Read the model definition and answer for the solid it produces. Units are mm, in the model's axes. A direction names the side the tool comes from. Give positions to 0.01 mm unless a question says otherwise; leave off trailing zeros. Order: outer loops, then holes, each group sorted by start corner. A loop starts at its lowest first (then second) coordinate and runs counter-clockwise, first axis right, second up. Notation, with made-up numbers: (22, 75.25) - (52, 75.25) arc R10 ccw to (52, 87.25) - close; hole circle Ø9 at (74.5, 77). An arc over 180 degrees is marked (long way). Write each question's results on one line, items separated by ' | '.
Autodesk Inventor part; units mm, degrees
ref_plane "Work Plane1" through (0, -27.5, 0) normal (1, 0, 0) x (0, 0, -1)
ref_plane "Work Plane2" through (-48.55, 0, 0) normal (0, 1, 0) x (1, 0, 0)
ref_plane "YZ Plane" through (0, 0, 0) normal (1, 0, 0) x (0, 1, 0)
sketch "Sketch1" plane through (0, 0, 0) normal (0, 0, 1) x (1, 0, 0)
  line L0 (-60, -27.5) -> (60, -27.5)
  line L1 (60, -27.5) -> (60, 27.5)
  line L2 (60, 27.5) -> (-60, 27.5)
  line L3 (-60, 27.5) -> (-60, -27.5)
  line L4 (-60, -27.5) -> (60, 27.5) construction
  line L5 (60, -27.5) -> (-60, 27.5) construction
  point P0 (0, 0)
  dimension "d0" = 120
  dimension "d1" = 55
extrude "Extrusion1" add sketch "Sketch1" against normal blind 4
sketch "Sketch2" plane through (60, -27.5, 0) normal (1, 0, 0) x (0, 0, -1)
  circle A0 centre (2, 2) radius 2
  line L0 (0, 0) -> (4, 0)
  line L1 (4, 55) -> (4, 0)
  circle A1 centre (2, 2) radius 1.25
  circle A2 centre (2, 53) radius 2
  line L2 (0, 55) -> (4, 55)
  circle A3 centre (2, 53) radius 1.25
  line L3 (0, 55) -> (0, 0)
  line L4 (0, 55) -> (4, 55)
  line L5 (4, 55) -> (4, 0)
  line L6 (4, 0) -> (0, 0)
  line L7 (0, 0) -> (0, 55)
  point P0 (0, 27.5)
  dimension "d4" = 4
  dimension "d5" = 2.5
  dimension "d6" = 4
  dimension "d7" = 2.5
extrude "Extrusion2" cut sketch "Sketch2" against normal blind 3.5 contours L1 L0 A0 | A0 L3 A2 L1 | A0 L0 L3 | A2 L2 L1 | L3 L2 A2
extrude "Extrusion3" cut sketch "Sketch2" against normal blind 25 contours A1
extrude "Extrusion4" cut sketch "Sketch2" against normal blind 25 contours A3
sketch "Sketch3" plane through (-60, -27.5, 0) normal (-1, 0, 0) x (0, 0, 1)
  circle A0 centre (-2, 2) radius 2
  circle A1 centre (-2, 53) radius 2
  line L0 (0, 0) -> (-4, 0)
  line L1 (-4, 0) -> (-4, 55)
  line L2 (0, 55) -> (-4, 55)
  line L3 (0, 55) -> (0, 0)
  line L4 (-4, 0) -> (0, 0)
  line L5 (0, 0) -> (0, 55)
  line L6 (0, 55) -> (-4, 55)
  line L7 (-4, 55) -> (-4, 0)
  circle A2 centre (-2, 2) radius 1.25
  circle A3 centre (-2, 2) radius 1.25
  circle A4 centre (-2, 53) radius 1.25
  circle A5 centre (-2, 53) radius 1.25
  point P0 (0, 27.5)
  dimension "d14" = 4
  dimension "d15" = 4
  dimension "d16" = 2.5
  dimension "d17" = 2.5
extrude "Extrusion5" cut sketch "Sketch3" against normal blind 3.5 contours L3 L0 A0 | A0 L1 A1 L3 | A0 L0 L1 | A1 L2 L3 | L1 L2 A1
extrude "Extrusion6" cut sketch "Sketch3" against normal blind 25 contours A4
extrude "Extrusion7" cut sketch "Sketch3" against normal blind 25 contours A2
sketch "Sketch4" plane through (0, 0, 0) normal (0, 0, 1) x (1, 0, 0)
  line L0 (-56.5, 27.5) -> (56.5, 27.5)
  line L1 (56.5, -27.5) -> (-56.5, -27.5)
  line L2 (-56.5, 27.5) -> (56.5, 27.5)
  line L3 (56.5, 27.5) -> (56.5, -27.5)
  line L4 (56.5, -27.5) -> (-56.5, -27.5)
  line L5 (-56.5, -27.5) -> (-56.5, 27.5)
  line L6 (-73.441, 25.5) -> (75.6749, 25.5) construction
  line L7 (-49.5, 37.9771) -> (-49.5, -42.6684) construction
  line L8 (-50.45, 28) -> (-48.55, 28)
  line L9 (-48.55, 28) -> (-48.55, 23)
  line L10 (-48.55, 23) -> (-50.45, 23)
  line L11 (-50.45, 23) -> (-50.45, 28)
  line L12 (-50.45, 28) -> (-48.55, 23) construction
  line L13 (-48.55, 28) -> (-50.45, 23) construction
  point P0 (0, 0)
  point P1 (-49.5, 25.5)
  dimension "d24" = 2
  dimension "d25" = 7
  dimension "d26" = 1.9
  dimension "d27" = 5
extrude "Extrusion8" cut sketch "Sketch4" against normal blind 25 contours L11 L8 L9 L0 | L0 L9 L10 L11
ref_plane "Work Plane1" through (0, -27.5, 0) normal (1, 0, 0) x (0, 0, -1)
ref_plane "Work Plane2" through (-48.55, 0, 0) normal (0, 1, 0) x (1, 0, 0)
mirror "Mirror1" about plane through (0, -27.5, 0) normal (1, 0, 0) of "Extrusion8"
mirror "Mirror3" about plane through (-48.55, 0, 0) normal (0, 1, 0) of "Extrusion8", "Mirror1"
sketch "Sketch5" plane through (0, 0, 0) normal (0, 0, 1) x (1, 0, 0)
  line L0 (-20.311, 26.3647) -> (47.689, 26.3647) construction
  line L1 (47.689, 26.3647) -> (47.689, -26.6353) construction
  line L2 (47.689, -26.6353) -> (-20.311, -26.6353) construction
  line L3 (-20.311, -26.6353) -> (-20.311, 26.3647) construction
  line L4 (34.689, 35.6432) -> (34.689, -53.7477) construction
  line L5 (-67.7221, 24) -> (59.2356, 24) construction
  line L6 (-64.2143, -24) -> (60.4803, -24) construction
  line L7 (-93.3625, 0) -> (86.1208, 0) construction
  circle A0 centre (34.689, 24) radius 2.5
  circle A1 centre (34.689, -24) radius 2.5
  line L8 (-15.0696, 19.4646) -> (-13.0566, 19.4646)
  line L9 (-13.0566, 19.4646) -> (-13.0566, -11.8201)
  line L10 (-13.0566, -11.8201) -> (-15.0696, -11.8201)
  line L11 (-15.0696, -11.8201) -> (-15.0696, 19.4646)
  circle A2 centre (34.689, 24) radius 0.75
  circle A3 centre (34.689, -24) radius 0.75
  point P0 (0, 0)
  dimension "d30" = 68
  dimension "d31" = 53
  dimension "d32" = 13
  dimension "d34" = 48
  dimension "d35" = 24
  dimension "d36" = 5
  dimension "d37" = 5
  dimension "d42" = 1.5
  dimension "d43" = 1.5
extrude "Extrusion9" add sketch "Sketch5" along normal blind 4 contours A0 | A1 | A2 | A3
extrude "Extrusion10" add sketch "Sketch5" along normal blind 4 contours L8 L9 L10 L11
sketch "Sketch6" plane through (34.689, 24, 4) normal (0, 0, 1) x (1, 0, 0)
  circle A0 centre (0, 0) radius 0.75
  circle A1 centre (0, -48.0486) radius 0.75
  point P0 (-34.689, -24)
  dimension "d44" = 1.5
  dimension "d45" = 1.5
extrude "Extrusion11" cut sketch "Sketch6" against normal blind 7
sketch "Sketch7" plane through (0, 0, 0) normal (0, 0, 1) x (1, 0, 0)
  line L0 (-56.5, -25.5) -> (-56.5, 25.5)
  line L1 (-56.5, 20) -> (-16.5, 20)
  line L2 (-16.5, 20) -> (-16.5, -20)
  line L3 (-16.5, -20) -> (-56.5, -20)
  line L4 (-56.5, -20) -> (-56.5, 20)
  line L5 (48.55, 27.5) -> (-48.55, 27.5)
  line L6 (-8.902, 20) -> (51.098, 20)
  line L7 (51.098, 20) -> (51.098, -20)
  line L8 (51.098, -20) -> (-8.902, -20)
  line L9 (-8.902, -20) -> (-8.902, 20)
  point P0 (0, 0)
  dimension "d48" = 40
  dimension "d49" = 40
  dimension "d50" = 7.5
  dimension "d51" = 60
extrude "Extrusion12" cut sketch "Sketch7" against normal blind 7
fillet "Fillet1" radius 2 6 edges at (-16.5, -20, -2) (-16.5, 20, -2) (-8.902, 20, -2) (-8.902, -20, -2) (51.098, 20, -2) (51.098, -20, -2)
properties part number "Drivercarrier"
(1) Each of these flat-tipped pins is pushed along its axis until it touches: pin 1 (1.2 mm diameter, centred on y = -8, z = -1.5, fed in from -X); pin 2 (2 mm diameter, centred on y = 2.5, z = 1.5, fed in from +X); pin 3 (2 mm diameter, centred on y = -8, z = -2, fed in from +X). Where does it stop, or does it pass through?
Conclusion:
pin 1: x = -16.5 | pin 2: x = -13.06 | pin 3: x = 56.5
(2) Consider probe 1 along Y at (x, z) = (-43, -2); probe 2 along X at (y, z) = (18, -3); probe 3 along Z at (x, y) = (44.5, -25.5). Determine where each line is inside the solid, lowest interval first. Write a range as [from, to].
Conclusion:
probe 1: [-27.5, -26.75], [-24.25, -20], [20, 24.25], [26.75, 27.5] | probe 2: [-16.5, -8.9], [51.1, 56.5] | probe 3: [-4, -3.25], [-0.75, 0]
(3) Section A-A (z = 1.5) is taken. Give the vertices of the cut face in (x, y).
Conclusion:
outline: (-15.07, -11.82) - (-13.06, -11.82) - (-13.06, 19.46) - (-15.07, 19.46) - close; circle Ø5 at (34.69, -24); circle Ø5 at (34.69, 24); hole circle Ø1.5 at (34.69, -24.05); hole circle Ø1.5 at (34.69, 24)
(4) Section B-B (x = 3) is taken. Give the vertices of the cut face in (y, z), plus the area to 3 significant figures.
Conclusion:
outline: (-27.5, -4) - (-20, -4) - (-20, 0) - (-27.5, 0) - close; (20, -4) - (27.5, -4) - (27.5, 0) - (20, 0) - close | area: 60.0 mm^2
(5) For faces 4 (the face through (-48.55, 24, -2)), 5 (the face through (-15.07, 4, 2)), 6 (the face through (-58.274, -27.452, -2.434)), 7 (the face through (-37, -20, -2)), 8 (the face through (21, 20, -2)), determine the directions among +Z, -Z, +X, -X, +Y, -Y from which every point of the face is accessible in a straight line to the end or side of a thin tool.
Conclusion:
face 4: +Z, -Z, +Y | face 5: +Z, -X, +Y, -Y | face 6: -X | face 7: +Z, -Z, -X | face 8: +Z, -Z
(6) The mould has two halves that part along Y. Classify faces 1 (the face through (-17.1, 19.43, -2.03)), 2 (the face through (50.45, 24, -2)), 3 (the face through (-54, -27.5, -2)): pulls with the +Y half, pulls with the -Y half, needs draft (parallel to the pull), parting line crosses it, or undercut.
Conclusion:
face 1: undercut | face 2: needs draft | face 3: pulls with the -Y half
